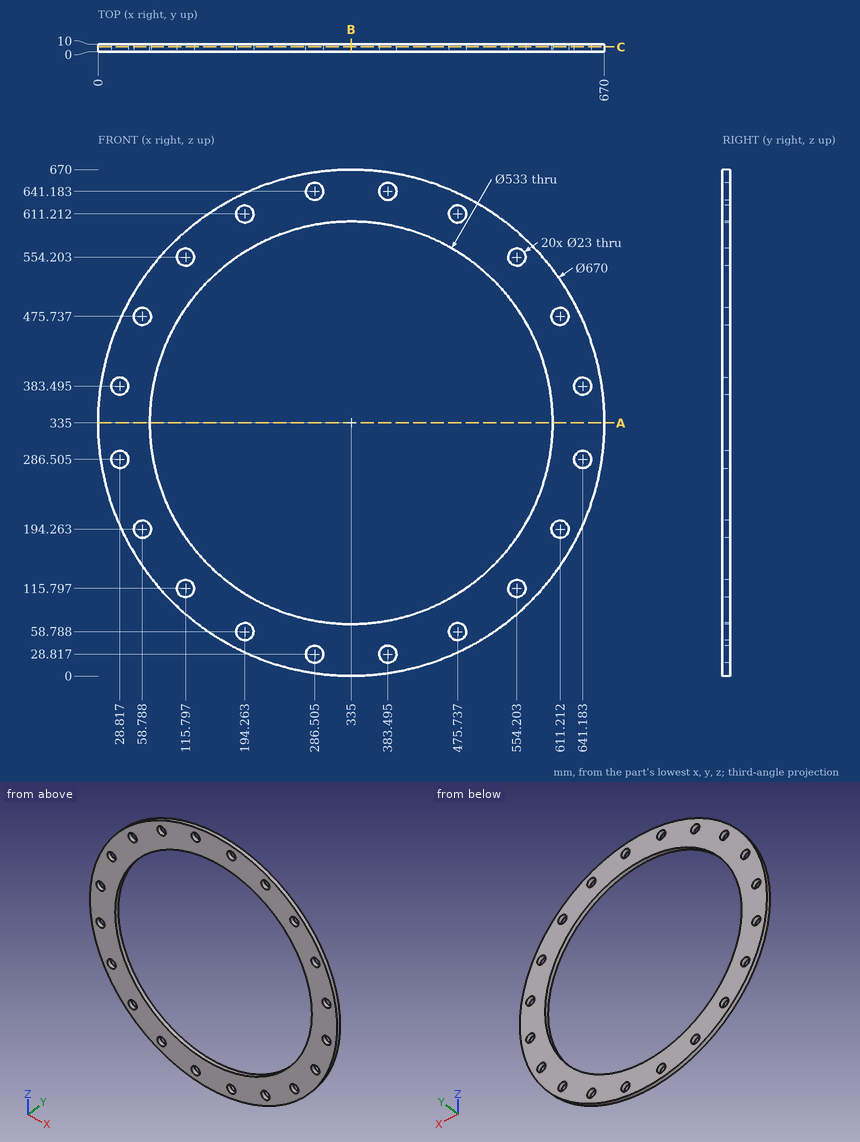
Study the drawing (mm; zero at the part's minimum x, y, z) and answer. Round coordinates to 2 decimals unless told otherwise and drop trailing zeros. Loops run counter-clockwise (first coordinate to the right, second up) from the corner with the lowest first, then second, coordinate; pieces in that order, holes last. Notation, with made-up numbers: (26.5, -30) -> (77.5, -30) arc R12 cw to (77.5, -20) -> close; hole circle Ø11 at (52.25, 42). An arc over 180 degrees is marked (long way). Write each question's results on one line, items separated by ' | '. Start each with the question number.
1. Section B-B (x = 335) is taken. Determine the outline of the cut face in (y, z).
2. Given pin 1 Ø2 at (x, y) = (410.5, 7.5) entering from -Z; pin 2 Ø3 at (y, z) = (6, 379) entering from -X; pin 3 Ø5 at (x, y) = (85, 3) entering from -Z, each flat-ended and moving along its own axis, determine where each tip first touches the part or whether it passes through.
3. Find the intervals of material crossed by probe 1 along Z at (x, y) = (53, 7) (1 decimal); probe 2 along Z at (x, y) = (327, 9.75) (1 decimal); probe 3 along Z at (x, y) = (68, 6.75) (1 decimal), in increasing order. Write a range as from..to.
4. Section C-C (y = 6.25) is taken. State how many separate pieces and enclosed holes the cut face has, plus the area to 3 significant figures.
5. Section A-A (z = 335) is taken. Determine the outline of the cut face in (x, y), plus the area to 3 significant figures.
Evaluation:
1) outline: (0, 0) -> (10, 0) -> (10, 68.5) -> (0, 68.5) -> close; (0, 601.5) -> (10, 601.5) -> (10, 670) -> (0, 670) -> close
2) pin 1: stops at z = 8.39 | pin 2: stops at x = 2.71 | pin 3: stops at z = 109.24
3) probe 1: z = 154.2..184.3, 204.2..465.8, 485.7..515.8 | probe 2: z = 0.1..68.6, 601.4..669.9 | probe 3: z = 132.7..187.4, 201.1..468.9, 482.6..537.3
4) separate pieces: 1 | enclosed holes: 21 | area: 121,000 mm2
5) outline: (0, 0) -> (68.5, 0) -> (68.5, 10) -> (0, 10) -> close; (601.5, 0) -> (670, 0) -> (670, 10) -> (601.5, 10) -> close | area: 1,370 mm2
